Source: CAD feature listing. Evaluate the final solid. Frame: model axes, mm. A direction names the side the tool comes from. Coordinates: 2 decimals unless noted, no trailing zeros. Write each loop counter-clockwise with the first axis right and the second up, starting at its lowest first coordinate (ties: lowest second). Pieces come first, ordered by that corner, then holes. Notation, with made-up numbers: (5.5, 32) - (11.5, 32) arc R9 cw to (11.5, 45) - close; hole circle Ø4 at (72.5, 38.25). An arc over 180 degrees is marked (long way). One line per item, written item: value.
from build123d import *

# Parameters (mm, degrees)
SKETCH_1_W          = 280
SKETCH_1_H          = 280
EXTRUDE_1_DEPTH     = 100
SKETCH_2_W          = 280
SKETCH_2_H          = 272
CUT_EXTRUDE_1_DEPTH = 2
SKETCH_3_W          = 280
SKETCH_3_H          = 4
CUT_EXTRUDE_2_DEPTH = 2
SKETCH_4_W          = 270
SKETCH_4_H          = 88
CUT_EXTRUDE_3_DEPTH = 278
SKETCH_6_W          = 260
SKETCH_6_H          = 232
CUT_EXTRUDE_7_DEPTH = 93
FILLET_4_R          = 2
FILLET_5_R          = 2
FILLET_6_R          = 2
SKETCH_8_W          = 19
SKETCH_8_H          = 4
EXTRUDE_2_DEPTH     = 278
FILLET_7_R          = 2


with BuildPart() as part:
    # 草图1 → 凸台-拉伸1 (new body)
    with BuildSketch(Plane(origin=(0, 0, 0), x_dir=(1, 0, 0), z_dir=(0, 1, 0))):
        Rectangle(SKETCH_1_W, SKETCH_1_H)
    extrude(amount=EXTRUDE_1_DEPTH)

    # 草图2 → 切除-拉伸1 (cut)
    with BuildSketch(Plane(origin=(0, 100, 0), x_dir=(1, 0, 0), z_dir=(0, 1, 0))):
        Rectangle(SKETCH_2_W, SKETCH_2_H)
    extrude(amount=-CUT_EXTRUDE_1_DEPTH, mode=Mode.SUBTRACT)

    # 草图3 → 切除-拉伸2 (cut)
    with BuildSketch(Plane.XZ):
        with Locations((0, 138)):
            Rectangle(SKETCH_3_W, SKETCH_3_H)
        with Locations((0, -138)):
            Rectangle(SKETCH_3_W, SKETCH_3_H)
    extrude(amount=-CUT_EXTRUDE_2_DEPTH, mode=Mode.SUBTRACT)

    # 草图4 → 切除-拉伸3 (cut)
    with BuildSketch(Plane(origin=(140, 0, 0), x_dir=(0, 0, -1), z_dir=(1, 0, 0))):
        with Locations((0, 49)):
            Rectangle(SKETCH_4_W, SKETCH_4_H)
    extrude(amount=-CUT_EXTRUDE_3_DEPTH, mode=Mode.SUBTRACT)

    # 草图6 → 切除-拉伸7 (cut)
    with BuildSketch(Plane(origin=(0, 98, 0), x_dir=(1, 0, 0), z_dir=(0, 1, 0))):
        with Locations((10, 0)):
            Rectangle(SKETCH_6_W, SKETCH_6_H)
    extrude(amount=-CUT_EXTRUDE_7_DEPTH, mode=Mode.SUBTRACT)

    # 圆角4
    fillet_4_edges = [part.edges().sort_by_distance(p)[0] for p in [
        (140, 51, -140),
        (140, 51, 140),
    ]]
    fillet(fillet_4_edges, radius=FILLET_4_R)

    # 圆角5
    fillet_5_edges = [part.edges().sort_by_distance(p)[0] for p in [
        (140, 98, 126),
        (140, 98, -126),
    ]]
    fillet(fillet_5_edges, radius=FILLET_5_R)

    # 圆角6
    fillet_6_edges = [part.edges().sort_by_distance(p)[0] for p in [
        (-120, 95.5, -116),
        (-120, 95.5, 116),
    ]]
    fillet(fillet_6_edges, radius=FILLET_6_R)

    # 草图8 → 凸台-拉伸2 (add)
    with BuildSketch(Plane(origin=(-138, 0, 0), x_dir=(0, 0, -1), z_dir=(1, 0, 0))):
        with Locations((-125.5, 49)):
            Rectangle(SKETCH_8_W, SKETCH_8_H)
        with Locations((125.5, 49)):
            Rectangle(SKETCH_8_W, SKETCH_8_H)
    extrude(amount=EXTRUDE_2_DEPTH)

    # 圆角7
    fillet_7_edges = [part.edges().sort_by_distance(p)[0] for p in [
        (-138, 72, 135),
        (-138, 26, -135),
        (1, 47, 135),
        (1, 51, 135),
        (1, 47, -135),
        (1, 51, -135),
        (1, 5, 135),
        (1, 93, 135),
        (1, 93, -135),
        (1, 5, -135),
        (-138, 26, 135),
        (-138, 93, 0),
        (-138, 72, -135),
        (-138, 5, 0),
    ]]
    fillet(fillet_7_edges, radius=FILLET_7_R)


solid = part.part
1) Material intervals for line 1 (Y direction, x = 30.5, z = 118.5); line 2 (Z direction, x = -99, y = 57); line 3 (Y direction, x = -98, z = -42), sorted ascending.
Values found:
line 1: 0 to 5, 47 to 51, 93 to 98
line 2: -140 to -135, 135 to 140
line 3: 0 to 5
2) Reachability of faces 1 (the flat face through (-125, 98, 9)), 2 (the flat face through (-3, 50, 140)), 3 (the flat face through (-1, 51, -124)) from +Z, -Z, +X, -X, +Y, -Y: full face, straight path, thin tool, end or side. Return the list, or none.
Values found:
face 1: +X, -X, +Y
face 2: +Z, +X, -X, +Y, -Y
face 3: +X
3) Section query A-A on y = 72. Output: boundary loops of the cut face in (x, z).
Values found:
outline: (-140, -140) - (138, -140) arc R2 ccw to (140, -138) - (140, -135) - (-136, -135) arc R2 cw to (-138, -133) - (-138, 133) arc R2 cw to (-136, 135) - (140, 135) - (140, 138) arc R2 ccw to (138, 140) - (-140, 140) - close
4) Draft query along Y for faces 4 (the flat face through (-2, 0, -2)), 5 (the flat face through (140, 2, 1)), 6 (the flat face through (4, 26, 135)). Return one class per face: released by +Y, released by -Y, zero draft, split by the parting line, or undercut.
Values found:
face 4: released by -Y
face 5: zero draft
face 6: undercut
5) Section query B-B on z = 34. Output: boundary loops of the cut face in (x, y).
Values found:
outline: (-140, 0) - (140, 0) - (140, 5) - (-136, 5) arc R2 cw to (-138, 7) - (-138, 91) arc R2 cw to (-136, 93) - (-120, 93) - (-120, 98) - (-140, 98) - close
6) Contact query for flat-ended pins moving along their axis: P1, Ø1.6, axis at x = 43, y = 0.5, coming from the +Z side; P2, Ø3, axis at x = -104.5, z = 49.5, coming from the +Y side; P3, Ø6, axis at y = 64.5, z = -53, coming from the +X side. Output: stop coordinate, or through.
Values found:
P1: z = 136
P2: y = 5
P3: x = -138
